Read the model definition and answer for the solid it produces. Units are mm, in the model's axes. Give positions to 0.01 mm unless a question says otherwise; leave off trailing zeros. Loops run counter-clockwise (first coordinate to the right, second up) from the corner with the lowest first, then second, coordinate; pieces in that order, holes last.
(1) Find section A-A, the plane y = 0. Write down the section's boundary in (x, z).
(2) Find section D-D, the plane x = 192. Write down the section's boundary in (y, z).
(3) Straight lines are drawn through the part: probe 1 along X at (y, z) = (-0.5, 4.55); probe 2 along Y at (x, z) = (-31.75, 3.95); probe 3 along Y at (x, z) = (31, 3.3). For each, find the intervals that lie inside material, in ascending order.
(4) Find section B-B, the plane z = 4.1. Write down the section's boundary in (x, y) (3 decimals), then the cut area to 3 significant figures.
(5) Find section C-C, the plane x = -31.75. Write down the section's boundary in (y, z), then the cut area to 3 significant figures.
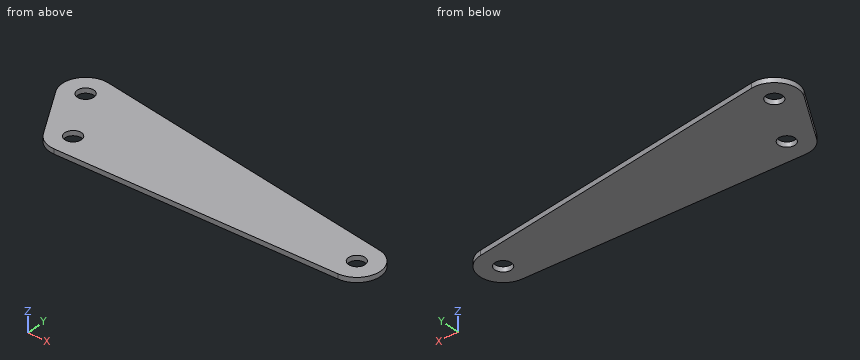
```python
from build123d import *

# Parameters (mm, degrees)
SKETCH1_R           = 8.5
BOSS_EXTRUDE1_DEPTH = 5
CUT_EXTRUDE1_DEPTH  = 6


with BuildPart() as part:
    # Sketch1 → Boss-Extrude1 (new body)
    with BuildSketch(Plane.XY):
        with BuildLine():
            Line((0, -31.75), (292.1, -31.75))
            ThreePointArc((292.1, -31.75), (323.737779408, -2.667098451), (297.415343146, 31.30191092))
            Line((297.415343146, 31.30191092), (-26.434656854, 86.29452406))
            ThreePointArc((-26.434656854, 86.29452406), (-57.815571461, 73.121277857), (-59.24630657, 39.11761314))
            Line((-59.24630657, 39.11761314), (-27.49630657, -15.875))
            ThreePointArc((-27.49630657, -15.875), (-15.875, -27.49630657), (0, -31.75))
        make_face()
        with Locations((-31.75, 54.99261314)):
            Circle(SKETCH1_R, mode=Mode.SUBTRACT)
        Circle(SKETCH1_R, mode=Mode.SUBTRACT)
        with Locations((292.1, 0)):
            Circle(SKETCH1_R, mode=Mode.SUBTRACT)
    extrude(amount=BOSS_EXTRUDE1_DEPTH)

    # Sketch2 → Cut-Extrude1 (cut, through all)
    with BuildSketch(Plane.XY.offset(5)):
        with BuildLine():
            Line((297.415343146, 31.30191092), (-26.434656854, 86.29452406))
            ThreePointArc((-26.434656854, 86.29452406), (-57.815571461, 73.121277857), (-59.24630657, 39.11761314))
            Line((-59.24630657, 39.11761314), (-27.49630657, -15.875))
            ThreePointArc((-27.49630657, -15.875), (-15.875, -27.49630657), (0, -31.75))
            Line((0, -31.75), (292.1, -31.75))
            ThreePointArc((292.1, -31.75), (323.737779408, -2.667098451), (297.415343146, 31.30191092))
        make_face()
        with BuildLine():
            Line((296.139660791, 23.789452299), (-27.710339209, 78.782065439))
            ThreePointArc((-27.710339209, 78.782065439), (-51.55983431, 68.770398325), (-52.647192993, 42.92761314))
            Line((-52.647192993, 42.92761314), (-20.897192993, -12.065))
            ThreePointArc((-20.897192993, -12.065), (-12.065, -20.897192993), (0, -24.13))
            Line((0, -24.13), (292.1, -24.13))
            ThreePointArc((292.1, -24.13), (316.14471235, -2.026994822), (296.139660791, 23.789452299))
        make_face(mode=Mode.SUBTRACT)
    extrude(amount=-CUT_EXTRUDE1_DEPTH, mode=Mode.SUBTRACT)


solid = part.part
```
Entries:
1. outline: (-27.86, 0) - (-8.5, 0) - (-8.5, 5) - (-27.86, 5) - close; (8.5, 0) - (283.6, 0) - (283.6, 5) - (8.5, 5) - close; (300.6, 0) - (316.23, 0) - (316.23, 5) - (300.6, 5) - close
2. outline: (-24.13, 0) - (41.47, 0) - (41.47, 5) - (-24.13, 5) - close
3. probe 1: x = -27.57 to -8.49, 8.49 to 283.61, 300.59 to 316.22
3. probe 2: y = 6.73 to 46.49, 63.49 to 79.12
3. probe 3: y = -24.13 to 68.81
4. outline: (-52.647, 42.928) - (-20.897, -12.065) arc R24.13 ccw to (0, -24.13) - (292.1, -24.13) arc R24.13 ccw to (296.14, 23.789) - (-27.71, 78.782) arc R24.13 ccw to start; hole circle Ø17 at (-31.75, 54.993); hole circle Ø17 at (0, 0); hole circle Ø17 at (292.1, 0)
4. area: 25,700 mm2
5. outline: (6.73, 0) - (46.49, 0) - (46.49, 5) - (6.73, 5) - close; (63.49, 0) - (79.12, 0) - (79.12, 5) - (63.49, 5) - close
5. area: 277 mm2
